```python
from build123d import *

# Parameters (mm, degrees)
SKETCH_1_W          = 40
SKETCH_1_H          = 14
EXTRUDE_2_DEPTH     = 3
SKETCH_2_R          = 1.6
CUT_EXTRUDE_1_DEPTH = 10
SKETCH_3_R          = 1.6
CUT_EXTRUDE_2_DEPTH = 87.585218138


with BuildPart() as part:
    # 草图1 → 凸台-拉伸2 (new body)
    with BuildSketch(Plane.XY):
        Polygon((0, 0), (0, 48), (72, 48), (72, 0), (56, 0), (16, 0), align=None)
        with Locations((36, 25)):
            Rectangle(SKETCH_1_W, SKETCH_1_H, mode=Mode.SUBTRACT)
    extrude(amount=EXTRUDE_2_DEPTH)

    # 草图2 → 切除-拉伸1 (cut)
    with BuildSketch(Plane(origin=(0, 0, 0), x_dir=(-1, 0, 0), z_dir=(0, 0, -1))):
        with Locations((-44, 12)):
            Circle(SKETCH_2_R)
        with Locations((-28, 12)):
            Circle(SKETCH_2_R)
        with Locations((-44, 40)):
            Circle(SKETCH_2_R)
        with Locations((-28, 40)):
            Circle(SKETCH_2_R)
        with Locations((-56, 40)):
            Circle(SKETCH_2_R)
        with Locations((-16, 40)):
            Circle(SKETCH_2_R)
        with Locations((-44, 5)):
            Circle(SKETCH_2_R)
        with Locations((-28, 5)):
            Circle(SKETCH_2_R)
    extrude(amount=-CUT_EXTRUDE_1_DEPTH, mode=Mode.SUBTRACT)

    # 草图3 → 切除-拉伸2 (cut, through all)
    with BuildSketch(Plane.XY.offset(3)):
        with Locations((67.5, 11)):
            Circle(SKETCH_3_R)
        with Locations((60.5, 11)):
            Circle(SKETCH_3_R)
        with Locations((4.5, 11)):
            Circle(SKETCH_3_R)
        with Locations((11.5, 11)):
            Circle(SKETCH_3_R)
    extrude(amount=-CUT_EXTRUDE_2_DEPTH, mode=Mode.SUBTRACT)


solid = part.part
```
Here's how the part is built. I have some questions about the finished solid (model axes, mm). A direction names the side the tool comes from. Give positions to 0.01 mm unless a question says otherwise; leave off trailing zeros. Loops run counter-clockwise (first coordinate to the right, second up) from the corner with the lowest first, then second, coordinate; pieces in that order, holes last. Notation, with made-up numbers: M 58.5,73.5 L 62.5,73.5 A28 ccw 62.5,99.5 Z; hole C 40,70.25 d6. An arc over 180 degrees is marked long. Use one line per item in the form item = value. Start each with the question number.
Q1. If we section it at D-D (x = 28): Write out the boundary of the cut face in (y, z), then the cut area to 3 significant figures.
Q2. Thinking about a two-plate mould opening in X: for faces 3 (the flat face through (0, 24, 1)), 4 (the flat face through (72, 24, 1)), 5 (the cylindrical face through (29.27, 4.03, 1.48)), 6 (the flat face through (35, 48, 1)), which applies, +X half, -X half, draft (parallel to the pull), parting line (faces both ways), or undercut?
Q3. Which directions (+Z, -Z, +X, -X, +Y, -Y) give clear straight access to the entire face, cutting with the end or side of a thin tool? Please do faces 1 (the flat face through (36, 18, 1)), 2 (the flat face through (37, 14, 0)).
Q4. If we section it at C-C (y = 40): Write out the boundary of the cut face in (x, z).
Q5. I need wall thicknesses on line 1 along Y through (x, z) = (28, 1.95); line 2 along Y through (x, z) = (33, 2.3); line 3 along X through (y, z) = (20, 1.6). Which ranges of each line are inside material? Lowest first, please.
Q6. If we section it at A-A (x = 46.5): Write out the boundary of the cut face in (y, z).
Q7. If we section it at B-B (z = 1.8): State how many separate pieces and enclosed holes the cut face has, then the cut area to 3 significant figures.
Taken from the geometry:
q1.outline = M 0,0 L 3.4,0 L 3.4,3 L 0,3 Z; M 6.6,0 L 10.4,0 L 10.4,3 L 6.6,3 Z; M 13.6,0 L 18,0 L 18,3 L 13.6,3 Z; M 32,0 L 38.4,0 L 38.4,3 L 32,3 Z; M 41.6,0 L 48,0 L 48,3 L 41.6,3 Z
q1.area = 73.2 mm^2
q2.face_3 = -X half
q2.face_4 = +X half
q2.face_5 = undercut
q2.face_6 = draft
q3.face_1 = +Z, -Z
q3.face_2 = -Z, +X, -X, +Y, -Y
q4.outline = M 0,0 L 14.4,0 L 14.4,3 L 0,3 Z; M 17.6,0 L 26.4,0 L 26.4,3 L 17.6,3 Z; M 29.6,0 L 42.4,0 L 42.4,3 L 29.6,3 Z; M 45.6,0 L 54.4,0 L 54.4,3 L 45.6,3 Z; M 57.6,0 L 72,0 L 72,3 L 57.6,3 Z
q5.line_1 = 0 to 3.4, 6.6 to 10.4, 13.6 to 18, 32 to 38.4, 41.6 to 48
q5.line_2 = 0 to 18, 32 to 48
q5.line_3 = 0 to 16, 56 to 72
q6.outline = M 0,0 L 18,0 L 18,3 L 0,3 Z; M 32,0 L 48,0 L 48,3 L 32,3 Z
q7.separate_pieces = 1
q7.enclosed_holes = 13
q7.area = 2,800 mm^2
